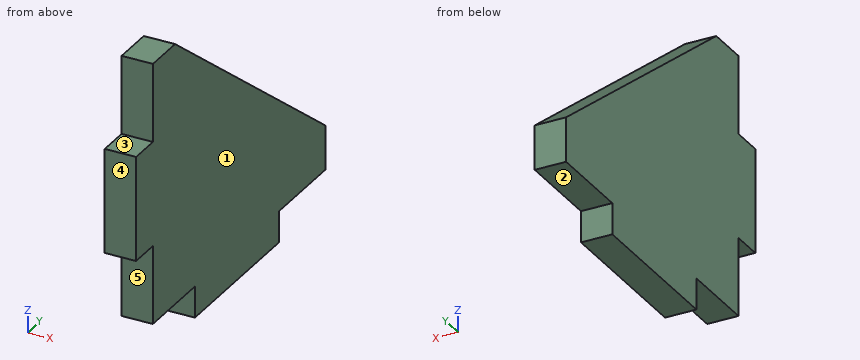
```python
from build123d import *

# Parameters (mm, degrees)
SKETCH1_W           = 6
SKETCH1_H           = 16.498322337
SKETCH1_H_2         = 30
SKETCH1_H_3         = 21
BOSS_EXTRUDE1_DEPTH = 50
SKETCH1_3_W         = 6
SKETCH1_3_H         = 30
BOSS_EXTRUDE2_DEPTH = 6
CUT_EXTRUDE1_DEPTH  = 6
CUT_EXTRUDE2_DEPTH  = 6


with BuildPart() as part:
    # Sketch1 → Boss-Extrude1 (new body)
    with BuildSketch(Plane.XY):
        with Locations((3, 19.249161169)):
            Rectangle(SKETCH1_W, SKETCH1_H)
        with Locations((3, -4)):
            Rectangle(SKETCH1_W, SKETCH1_H_2)
        with Locations((3, -29.5)):
            Rectangle(SKETCH1_W, SKETCH1_H_3)
    extrude(amount=BOSS_EXTRUDE1_DEPTH)

    # Sketch1_3 → Boss-Extrude2 (add)
    with BuildSketch(Plane.XY):
        with Locations((3, -4)):
            Rectangle(SKETCH1_3_W, SKETCH1_3_H)
    extrude(amount=-BOSS_EXTRUDE2_DEPTH)

    # Sketch2 → Cut-Extrude1 (cut)
    with BuildSketch(Plane.ZY):
        Polygon((0, -34), (15, -34), (15, -40), (35, -40), (35, -34), (50, -34), (50, -43.159116413), (0, -43.159116413), align=None)
    extrude(amount=-CUT_EXTRUDE1_DEPTH, mode=Mode.SUBTRACT)

    # Sketch3 → Cut-Extrude2 (cut)
    with BuildSketch(Plane.ZY):
        Polygon((8.542523628, 27.498322337), (50, -26.085899573), (50, 27.498322337), align=None)
    extrude(amount=-CUT_EXTRUDE2_DEPTH, mode=Mode.SUBTRACT)


solid = part.part
```
Could you check a few things on this model? Use its own coordinates, in mm. Face numbers are marked on the shaded views. A direction names the side the tool comes from. Round coordinates to 2 decimals unless told otherwise and drop trailing zeros. Loops run counter-clockwise (first coordinate to the right, second up) from the corner with the lowest first, then second, coordinate; pieces in that order, holes last. Notation, with made-up numbers: (9.25, -14) - (47.25, -14) arc R20 ccw to (47.25, -2) - close; hole circle Ø4 at (77, 8). An arc over 180 degrees is marked (long way). Use CSV: the item, a comma, the result in double quotes.
Item 1: For the marked faces 1, 2, 3, 4 and 5, which set-ups out of +Z, -Z, +X, -X, +Y, -Y let a thin tool reach every point of the face, with its end or its side?
Here are the results:
face 1,"+Z, -Z, +X, +Y, -Y"
face 2,"-Z, +X, -X, +Y"
face 3,"+Z, +X, -X, -Y"
face 4,"+Z, -Z, +X, -X, -Y"
face 5,"-Z, +X, -X, -Y"
Item 2: If we section it at A-A on x = 1.25: List the corners of the cut face in (y, z) for me, then the cut area to 3 significant figures.
Here are the results:
outline,"(-40, 15) - (-34, 15) - (-34, 0) - (-19, 0) - (-19, -6) - (11, -6) - (11, 0) - (27.5, 0) - (27.5, 8.54) - (-26.09, 50) - (-34, 50) - (-34, 35) - (-40, 35) - close"
area,"2,260 mm²"
Item 3: Will these pins go through, and if not, where does the flat tip stop? pin 1 (12 mm diameter, centred on y = -23, z = 31, fed in from -X); pin 2 (3 mm diameter, centred on x = 4, y = -36.5, fed in from -Z); pin 3 (1.8 mm diameter, centred on x = 3.5, y = -26, fed in from -Z); pin 4 (3 mm diameter, centred on x = 1, y = 13.5, fed in from +Z).
Here are the results:
pin 1,"stops at x = 0"
pin 2,"stops at z = 15"
pin 3,"stops at z = 0"
pin 4,"stops at z = 20.53"
Item 4: If we section it at C-C on y = 4.5: List the corners of the cut face in (x, z) for me.
Here are the results:
outline,"(0, -6) - (6, -6) - (6, 26.34) - (0, 26.34) - close"
Item 5: If we section it at B-B on z = 7: List the corners of the cut face in (x, y) for me.
Here are the results:
outline,"(0, -34) - (6, -34) - (6, 27.5) - (0, 27.5) - close"
Item 6: I need wall thicknesses on L1, parallel to Y at x = 2.35, z = 5; L2, parallel to Z at x = 4.95, y = -29; L3, parallel to Z at x = 1.8, y = -20. Which ranges of each line are inside material? Lowest first, please. Write a range as [from, to].
Here are the results:
L1,"y = [-34, 27.5]"
L2,"z = [0, 50]"
L3,"z = [0, 45.29]"
